The listing builds one solid part. Answer for the finished solid, in the listing's coordinates (mm). A direction names the side the tool comes from. Round coordinates to 2 decimals unless told otherwise and drop trailing zeros. Order: outer loops, then holes, each group sorted by start corner. A loop starts at its lowest first (then second) coordinate and runs counter-clockwise, first axis right, second up. Notation, with made-up numbers: (-27.5, 82) -> (23.5, 82) arc R30 cw to (23.5, 121) -> close; hole circle Ø1 at (-40, 13). An arc over 180 degrees is marked (long way). Answer in a Markdown table with one row per item. Add a question column.
```python
from build123d import *

# Parameters (mm, degrees)
SKETCH1_R           = 21
SKETCH1_R_2         = 14
BOSS_EXTRUDE1_DEPTH = 180
SKETCH3_W           = 126
SKETCH3_H           = 18
BOSS_EXTRUDE3_DEPTH = 67.5
SKETCH4_W           = 36
SKETCH4_H           = 6
CUT_EXTRUDE1_DEPTH  = 135
SKETCH5_R           = 15
SKETCH5_R_2         = 7.5
BOSS_EXTRUDE4_DEPTH = 7
FILLET1_R           = 4
BOSS_EXTRUDE5_START = -15
BOSS_EXTRUDE5_DEPTH = 15
BOSS_EXTRUDE6_START = 15
BOSS_EXTRUDE6_DEPTH = 15
CUT_EXTRUDE2_START  = -49
SKETCH9_R           = 7.5
CUT_EXTRUDE2_DEPTH  = 49


with BuildPart() as part:
    # Sketch1 → Boss-Extrude1 (new body)
    with BuildSketch(Plane.XY):
        with Locations(Location((0, 0, 0), (0, 0, 180))):
            Circle(SKETCH1_R)
        with Locations(Location((0, 0, 0), (0, 0, 180))):
            Circle(SKETCH1_R_2, mode=Mode.SUBTRACT)
    extrude(amount=BOSS_EXTRUDE1_DEPTH)



with BuildPart() as body_2:
    # Sketch3 → Boss-Extrude3 (new, symmetric)
    with BuildSketch(Plane(origin=(0, 0, 90), x_dir=(-1, 0, 0), z_dir=(0, 0, -1))):
        with Locations((0, -96)):
            Rectangle(SKETCH3_W, SKETCH3_H)
    extrude(amount=BOSS_EXTRUDE3_DEPTH, both=True)

    # Sketch4 → Cut-Extrude1 (cut)
    with BuildSketch(Plane(origin=(63, 0, 0), x_dir=(0, 0, -1), z_dir=(1, 0, 0))):
        with Locations((-127.5, -102)):
            Rectangle(SKETCH4_W, SKETCH4_H)
    extrude(amount=-CUT_EXTRUDE1_DEPTH, mode=Mode.SUBTRACT)

    # Sketch5 → Boss-Extrude4 (add)
    with BuildSketch(Plane(origin=(0, -87, 0), x_dir=(1, 0, 0), z_dir=(0, 1, 0))):
        with Locations(Location((0, -76.5, 0), (0, 0, 90))):
            Circle(SKETCH5_R)
        with Locations(Location((0, -76.5, 0), (0, 0, 270))):
            Circle(SKETCH5_R_2, mode=Mode.SUBTRACT)
    extrude(amount=BOSS_EXTRUDE4_DEPTH)

    # Fillet1
    fillet1_edges = [body_2.edges().sort_by_distance(p)[0] for p in [
        (0, -87, 91.5),
    ]]
    fillet(fillet1_edges, radius=FILLET1_R)


with BuildPart() as part_1:
    add(part.part)

    add(body_2.part)  # Boss-Extrude5 merges body 2
    # Sketch6 → Boss-Extrude5 (add)
    with BuildSketch(Plane.XY.offset(145).offset(BOSS_EXTRUDE5_START)):
        with BuildLine():
            Line((-21, 0), (-21, -87))
            Line((-21, -87), (63, -87))
            Line((63, -87), (19.088523196, 8.753758176))
            ThreePointArc((19.088523196, 8.753758176), (4.48001188, -20.51656632), (-21, 0))
        make_face()
    extrude(amount=BOSS_EXTRUDE5_DEPTH)

    # Sketch8 → Boss-Extrude6 (add)
    with BuildSketch(Plane(origin=(0, 0, 49), x_dir=(-1, 0, 0), z_dir=(0, 0, -1)).offset(BOSS_EXTRUDE6_START)):
        with BuildLine():
            Line((0, -21), (-15.31737287, -21))
            ThreePointArc((-15.31737287, -21), (-20.659650317, -22.546594078), (-24.349460831, -26.707985664))
            Line((-24.349460831, -26.707985664), (-53, -87))
            Line((-53, -87), (-63, -87))
            Line((-63, -87), (-19.088523196, 8.753758176))
            ThreePointArc((-19.088523196, 8.753758176), (-17.675249952, -11.339556391), (0, -21))
        make_face()
    extrude(amount=-BOSS_EXTRUDE6_DEPTH)

    # Sketch9 → Cut-Extrude2 (cut)
    with BuildSketch(Plane(origin=(0, -87, 0), x_dir=(1, 0, 0), z_dir=(0, 1, 0)).offset(CUT_EXTRUDE2_START)):
        with Locations(Location((0, -76.5, 0), (0, 0, 270))):
            Circle(SKETCH9_R)
    extrude(amount=CUT_EXTRUDE2_DEPTH, mode=Mode.SUBTRACT)


solid = part_1.part
```
1. The part is cut by section D-D (z = 134.5). Give the vertices of the cut face in (x, y), then the cut area to 3 significant figures.
2. The mould has two halves that part along Y. Classify faces 4 (the flat face through (41.35, -39.79, 41.4)), 5 (the flat face through (11, -49, 130)), 6 (the cylindrical face through (-19.4, 8.04, 88.74)), 7 (the flat face through (-21, -43, 137)): released by +Y, released by -Y, zero draft, split by the parting line, or undercut.
3. The part is cut by section C-C (y = -68). Give the vertices of the cut face in (x, z), then the cut area to 3 significant figures.
4. Each of these flat-tipped pins is pushed along its axis until it touches: pin 1 (16.5 mm diameter, centred on y = -25, z = 136.5, fed in from -X); pin 2 (6.5 mm diameter, centred on x = -1, y = -102, fed in from +Z); pin 3 (3 mm diameter, centred on x = 34, z = 97.5, fed in from +Y); pin 4 (2 mm diameter, centred on x = 13, y = 4, fed in from +Z). Where does it stop, or does it pass through?
5. Straight lines are drawn through the part: line 1 along Y through (x, z) = (0, 95); line 2 along Y through (x, z) = (0, 113); line 3 along X through (y, z) = (-98, 76). For each, find the intervals that lie inside material, in ascending order.
6. The part is cut by section B-B (z = 153.5). Give the vertices of the cut face in (x, y), then the cut area to 3 significant figures.
7. For faces 1 (the flat face through (1, -102, 109.5)), 2 (the flat face through (8, -21, 41)), 3 (the flat face through (1, -96, 22.5)), determine the directions among +Z, -Z, +X, -X, +Y, -Y from which every point of the face is accessible in a straight line to the end or side of a thin tool.
8. The part is cut by section A-A (z = 76.5). Give the vertices of the cut face in (x, y).
Report:
| question | item | result |
|---|---|---|
| 1 | outline | (-63, -99) -> (63, -99) -> (63, -87) -> (19.09, 8.75) arc R21 ccw to (-21, 0) -> (-21, -87) -> (-63, -87) -> close; hole circle Ø28 at (0, 0) |
| 1 | area | 7,170 mm^2 |
| 2 | face 4 | released by +Y |
| 2 | face 5 | undercut |
| 2 | face 6 | undercut |
| 2 | face 7 | zero draft |
| 3 | outline | (-21, 130) -> (54.29, 130) -> (54.29, 145) -> (-21, 145) -> close; (43.97, 34) -> (54.29, 34) -> (54.29, 49) -> (43.97, 49) -> close |
| 3 | area | 1,280 mm^2 |
| 4 | pin 1 | stops at x = -21 |
| 4 | pin 2 | stops at z = 157.5 |
| 4 | pin 3 | stops at y = -87 |
| 4 | pin 4 | stops at z = 180 |
| 5 | line 1 | y = -105 to -86.97, -21 to -14, 14 to 21 |
| 5 | line 2 | y = -99 to -87, -21 to -14, 14 to 21 |
| 5 | line 3 | x = -63 to -7.48, 7.48 to 63 |
| 6 | outline | (-63, -105) -> (63, -105) -> (63, -87) -> (-63, -87) -> close; circle Ø42 at (0, 0); hole circle Ø28 at (0, 0) |
| 6 | area | 3,040 mm^2 |
| 7 | face 1 | +X, -X, -Y |
| 7 | face 2 | -Z, -X |
| 7 | face 3 | -Z, +X, -X, -Y |
| 8 | outline | (-63, -105) -> (-7.5, -105) -> (-7.5, -80) -> (-15, -80) -> (-15, -83) arc R4 cw to (-19, -87) -> (-63, -87) -> close; circle Ø42 at (0, 0); (7.5, -105) -> (63, -105) -> (63, -87) -> (19, -87) arc R4 cw to (15, -83) -> (15, -80) -> (7.5, -80) -> close; hole circle Ø28 at (0, 0) |
